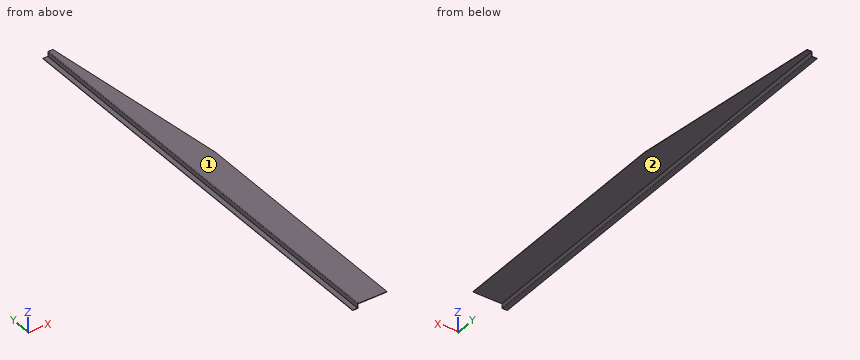
```python
from build123d import *

# Parameters (mm, degrees)
BRIDA_BASE4_DEPTH          = 1810
CORTAR_EXTRUIR1_DEPTH      = 1812.921593226
CORTAR_EXTRUIR1_DEPTH_BACK = 1812.921593226
CORTAR_EXTRUIR2_DEPTH      = 1.9
CORTAR_EXTRUIR3_DEPTH      = 1812.899624703
CORTAR_EXTRUIR3_DEPTH_BACK = 1812.899624703
CROQUIS22_W                = 55.247943396
CROQUIS22_H                = 1.9


# Read off the part's stored shape, not the designer's step: Cortar-Extruir2
# Sheet-metal steps are written as plain solids
with BuildPart() as part:
    # Croquis1 → Brida base4 (new body)
    with BuildSketch(Plane(origin=(0, 0, 0), x_dir=(1, 0, 0), z_dir=(0, 1, 0))):
        with BuildLine():
            Line((60.5, 0), (-57.8634, 0))
            ThreePointArc((-57.8634, 0), (-59.727757739, 0.772242261), (-60.5, 2.6366))
            Line((-60.5, 2.6366), (-60.5, 19.2634))
            ThreePointArc((-60.5, 19.2634), (-60.715745145, 19.784254855), (-61.2366, 20))
            Line((-61.2366, 20), (-80.5, 20))
            Line((-80.5, 20), (-80.5, 21.9))
            Line((-80.5, 21.9), (-61.2366, 21.9))
            ThreePointArc((-61.2366, 21.9), (-59.372242261, 21.127757739), (-58.6, 19.2634))
            Line((-58.6, 19.2634), (-58.6, 2.6366))
            ThreePointArc((-58.6, 2.6366), (-58.384254855, 2.115745145), (-57.8634, 1.9))
            Line((-57.8634, 1.9), (60.5, 1.9))
            Line((60.5, 1.9), (60.5, 0))
        make_face()
    extrude(amount=BRIDA_BASE4_DEPTH)

    # Croquis19 → Cortar-Extruir1 (cut, two sides: drawn at the far end of the back side and taken through both)
    with BuildSketch(Plane.XY.offset(-CORTAR_EXTRUIR1_DEPTH_BACK)):
        Polygon((60.5, 1000), (-39.5, 1810), (-39.5, 1900.089959651), (60.5, 1900.089959651), align=None)
    extrude(amount=CORTAR_EXTRUIR1_DEPTH + CORTAR_EXTRUIR1_DEPTH_BACK, mode=Mode.SUBTRACT)

    # Cortar-Extruir2 outline → Cortar-Extruir2 (cut)
    with BuildSketch(Plane(origin=(0, 0, 0), x_dir=(1, 0, 0), z_dir=(0, 1, 0))):
        with BuildLine():
            Line((-57.8634, 0), (-57.8634, 1.9))
            ThreePointArc((-57.8634, 1.9), (-58.384254855, 2.115745145), (-58.6, 2.6366))
            Line((-58.6, 2.6366), (-58.6, 19.2634))
            ThreePointArc((-58.6, 19.2634), (-59.372242261, 21.127757739), (-61.2366, 21.9))
            Line((-61.2366, 21.9), (-80.5, 21.9))
            Line((-80.5, 21.9), (-80.5, 20))
            Line((-80.5, 20), (-61.2366, 20))
            ThreePointArc((-61.2366, 20), (-60.715745145, 19.784254855), (-60.5, 19.2634))
            Line((-60.5, 19.2634), (-60.5, 2.6366))
            ThreePointArc((-60.5, 2.6366), (-59.727757739, 0.772242261), (-57.8634, 0))
        make_face()
    extrude(amount=CORTAR_EXTRUIR2_DEPTH, mode=Mode.SUBTRACT)

    # Croquis22 → Cortar-Extruir3 (cut, two sides: drawn at the far end of the back side and taken through both)
    with BuildSketch(Plane.XY.offset(-20).offset(-CORTAR_EXTRUIR3_DEPTH_BACK)):
        with Locations((-52.876028302, 1809.05)):
            Rectangle(CROQUIS22_W, CROQUIS22_H)
    extrude(amount=CORTAR_EXTRUIR3_DEPTH + CORTAR_EXTRUIR3_DEPTH_BACK, mode=Mode.SUBTRACT)


solid = part.part
```
Can you work these out from the model? Positions are in its coordinate system, mm. Face numbers are marked on the shaded views. A direction names the side the tool comes from. Coordinates: 2 decimals unless noted, no trailing zeros. Loops run counter-clockwise (first coordinate to the right, second up) from the corner with the lowest first, then second, coordinate; pieces in that order, holes last. Notation, with made-up numbers: (-23.5, 62) -> (2.5, 62) arc R14 ccw to (2.5, 79) -> close; hole circle Ø9 at (-6, 50). An arc over 180 degrees is marked (long way). Put each result on its own line as item: value. Start each with the question number.
Q1. I want a section at A-A (y = 331.5). Write out the boundary of the cut face in (x, z).
Q2. I want a section at B-B (x = 2.5). Write out the boundary of the cut face in (y, z), plus the area to 3 significant figures.
Q3. I'm going to push flat-ended pins straight in: P1, Ø5, axis at y = 1138, z = -10, coming from the +X side; P2, Ø1, axis at x = -59, y = 577.5, coming from the +Z side; P3, Ø0.6, axis at y = 1.5, z = -1, coming from the -X side; P4, Ø8, axis at x = -66.5, z = -14.5, coming from the -Y side. Where does each tip first touch, or does it pass through?
Q4. If I drill on line 1 (X direction, y = 625, z = -11.75); line 2 (Z direction, x = -4.5, y = 656.5); line 3 (Z direction, x = -75, y = 617), over which ranges is the centre line in solid material (lowest first)? Write a range as [from, to].
Q5. For the marked faces 1 and 2, which set-ups out of +Z, -Z, +X, -X, +Y, -Y let a thin tool reach every point of the face, with its end or its side?
Q6. I want a section at C-C (z = -10.75). Write out the boundary of the cut face in (x, y).
Q7. I want a section at D-D (y = 1276). Write out the boundary of the cut face in (x, z).
Taken from the geometry:
1. outline: (-80.5, -21.9) -> (-61.24, -21.9) arc R2.64 ccw to (-58.6, -19.26) -> (-58.6, -2.64) arc R0.74 cw to (-57.86, -1.9) -> (60.5, -1.9) -> (60.5, 0) -> (-57.86, 0) arc R2.64 ccw to (-60.5, -2.64) -> (-60.5, -19.26) arc R0.74 cw to (-61.24, -20) -> (-80.5, -20) -> close
2. outline: (0, -1.9) -> (1469.8, -1.9) -> (1469.8, 0) -> (0, 0) -> close
2. area: 2,790 mm2
3. P1: stops at x = -58.6
3. P2: stops at z = -0.08
3. P3: stops at x = -57.86
3. P4: passes through
4. line 1: x = [-60.5, -58.6]
4. line 2: z = [-1.9, 0]
4. line 3: z = [-21.9, -20]
5. face 1: +Z, +X, -X, +Y, -Y
5. face 2: -Z, +X, +Y, -Y
6. outline: (-60.5, 1.9) -> (-58.6, 1.9) -> (-58.6, 1808.1) -> (-60.5, 1808.1) -> close
7. outline: (-80.5, -21.9) -> (-61.24, -21.9) arc R2.64 ccw to (-58.6, -19.26) -> (-58.6, -2.64) arc R0.74 cw to (-57.86, -1.9) -> (26.43, -1.9) -> (26.43, 0) -> (-57.86, 0) arc R2.64 ccw to (-60.5, -2.64) -> (-60.5, -19.26) arc R0.74 cw to (-61.24, -20) -> (-80.5, -20) -> close
